The figure shows three views and two pictorial views of one solid part (mm, origin at its lowest corner). Answer the questions. A direction names the side the tool comes from. Give positions to 0.01 mm unless a question says otherwise; leave off trailing zeros. Write each loop counter-clockwise with the first axis right and the second up, starting at its lowest first coordinate (ties: lowest second). Pieces come first, ordered by that corner, then holes. Notation, with made-up numbers: (26.5, 24) -> (68.5, 24) arc R17 cw to (68.5, 56) -> close; hole circle Ø8 at (79.25, 43.5). An arc over 180 degrees is marked (long way). Answer as CSV lines item,"result". Start each with the question number.
1. The part is cut by section B-B, the plane y = 18.25. Determine the outline of the cut face in (x, z).
2. The part is cut by section D-D, the plane x = 14.5. Determine the outline of the cut face in (y, z) (1 decimal).
3. Find the intervals of material crossed by line 1 (Y direction, x = 8.89, z = 2.3) (1 decimal); line 2 (X direction, y = 13.75, z = 1) (1 decimal); line 3 (X direction, y = 22.25, z = 2.3), in increasing order.
4. A tool of negligible diameter and unlimited length cuts with its end or side. For the marked faces 1 and 2, from which of +Z, -Z, +X, -X, +Y, -Y can it reach the whole face along a straight path? Write none if from no direction.
5. The part is cut by section A-A, the plane z = 4.25. Determine the outline of the cut face in (x, y) (1 decimal).
6. The part is cut by section C-C, the plane x = 8.89. Determine the outline of the cut face in (y, z) (1 decimal).
7. Given pin 1 (2 mm diameter, centred on y = 21, z = 1.5, fed in from +X); pin 2 (1.5 mm diameter, centred on x = 17, z = 1.5, fed in from +Y) (3 decimals); pin 3 (2.5 mm diameter, centred on x = 19.5, z = 3.5, fed in from -Y) (3 decimals); pin 4 (1 mm diameter, centred on x = 20.5, y = 20, fed in from -Z), each flat-ended and moving along its own axis, determine where each tip first touches the part or whether it passes through.
8. For a pull along X with two mould halves and no side action, classify the marked faces 3, 4 and 5 as pulls with the +X half, pulls with the -X half, needs draft (parallel to the pull), parting line crosses it, or undercut.
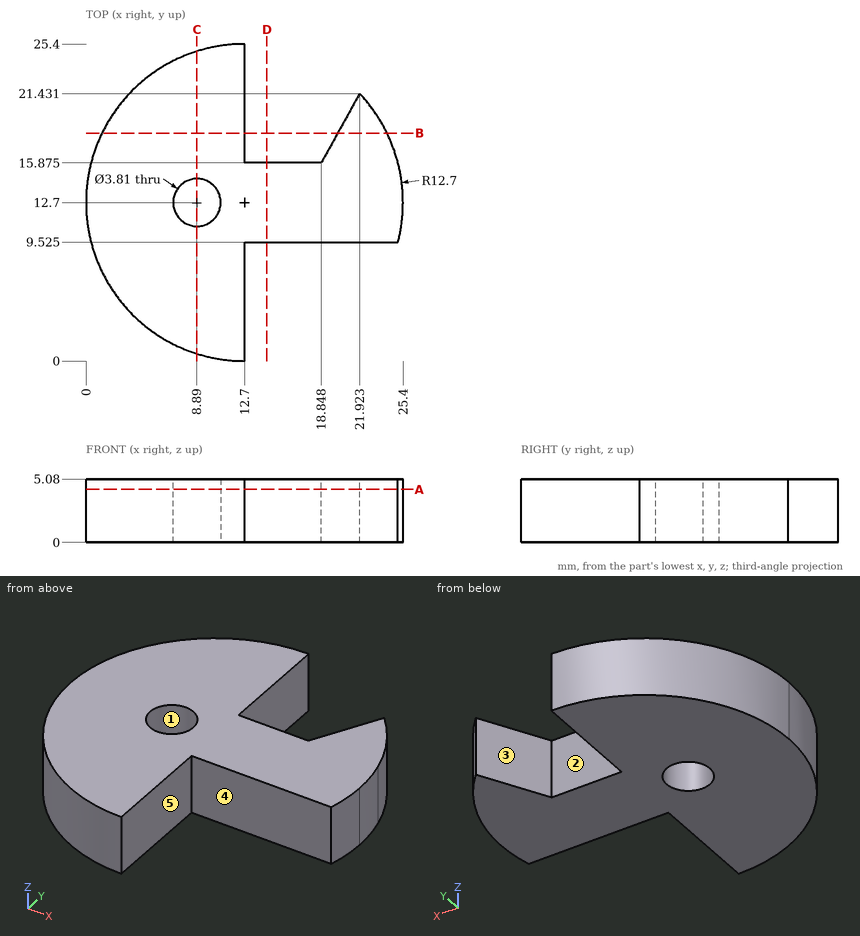
Results found:
1,outline,"(1.28, 0) -> (12.7, 0) -> (12.7, 5.08) -> (1.28, 5.08) -> close; (20.16, 0) -> (24.12, 0) -> (24.12, 5.08) -> (20.16, 5.08) -> close"
2,outline,"(9.5, 0) -> (15.9, 0) -> (15.9, 5.1) -> (9.5, 5.1) -> close"
3,line 1,"y = 0.6 to 10.8, 14.6 to 24.8"
3,line 2,"x = 0 to 7.3, 10.5 to 25.4"
3,line 3,"x = 4.33 to 12.7"
4,face 1,"+Z, -Z"
4,face 2,"+Z, -Z, +Y"
5,outline,"(12.7, 0) -> (12.7, 9.5) -> (25, 9.5) arc R12.7 ccw to (21.9, 21.4) -> (18.8, 15.9) -> (12.7, 15.9) -> (12.7, 25.4) arc R12.7 ccw to start; hole circle Ø3.8 at (8.9, 12.7)"
6,outline,"(0.6, 0) -> (10.8, 0) -> (10.8, 5.1) -> (0.6, 5.1) -> close; (14.6, 0) -> (24.8, 0) -> (24.8, 5.1) -> (14.6, 5.1) -> close"
7,pin 1,"stops at x = 23.09"
7,pin 2,"stops at y = 15.875"
7,pin 3,"stops at y = 9.525"
7,pin 4,"passes through"
8,face 3,"undercut"
8,face 4,"needs draft"
8,face 5,"pulls with the +X half"
